The listing builds one solid part. Answer for the finished solid, in the listing's coordinates (mm). A direction names the side the tool comes from. Coordinates: 2 decimals unless noted, no trailing zeros. Write each loop counter-clockwise with the first axis right and the second up, starting at its lowest first coordinate (ties: lowest second). Pieces come first, ordered by that corner, then holes.
```python
from build123d import *

# Parameters (mm, degrees)
SKETCH_1_W          = 31.8
SKETCH_1_H          = 15.8
EXTRUDE_1_DEPTH     = 9.6
SKETCH_2_R          = 2.4
EXTRUDE_4_DEPTH     = 1.7
SKETCH_3_R          = 2.5
CUT_EXTRUDE_1_DEPTH = 1.8


with BuildPart() as part:
    # Эскиз1 → Бобышка-Вытянуть1 (new body)
    with BuildSketch(Plane(origin=(0, 0, 0), x_dir=(1, 0, 0), z_dir=(0, 1, 0))):
        with Locations((15.9, 7.9)):
            Rectangle(SKETCH_1_W, SKETCH_1_H)
    extrude(amount=EXTRUDE_1_DEPTH)

    # Эскиз2 → Бобышка-Вытянуть4 (add)
    with BuildSketch(Plane.XZ):
        with Locations((27.9, -3.9)):
            Circle(SKETCH_2_R)
        with Locations((19.9, -3.9)):
            Circle(SKETCH_2_R)
        with Locations((11.9, -3.9)):
            Circle(SKETCH_2_R)
        with Locations((3.9, -3.9)):
            Circle(SKETCH_2_R)
        with Locations((19.9, -11.9)):
            Circle(SKETCH_2_R)
        with Locations((11.9, -11.9)):
            Circle(SKETCH_2_R)
        with Locations((3.9, -11.9)):
            Circle(SKETCH_2_R)
        with Locations((27.9, -11.9)):
            Circle(SKETCH_2_R)
    extrude(amount=EXTRUDE_4_DEPTH)

    # Эскиз3 → Вырез-Вытянуть1 (cut)
    with BuildSketch(Plane(origin=(0, 9.6, 0), x_dir=(1, 0, 0), z_dir=(0, 1, 0))):
        with Locations((27.9, 3.9)):
            Circle(SKETCH_3_R)
        with Locations((19.9, 3.9)):
            Circle(SKETCH_3_R)
        with Locations((11.9, 3.9)):
            Circle(SKETCH_3_R)
        with Locations((3.9, 3.9)):
            Circle(SKETCH_3_R)
        with Locations((19.9, 11.9)):
            Circle(SKETCH_3_R)
        with Locations((11.9, 11.9)):
            Circle(SKETCH_3_R)
        with Locations((3.9, 11.9)):
            Circle(SKETCH_3_R)
        with Locations((27.9, 11.9)):
            Circle(SKETCH_3_R)
    extrude(amount=-CUT_EXTRUDE_1_DEPTH, mode=Mode.SUBTRACT)


solid = part.part
```
(1) Section C-C, the plane x = 4.5 is taken. Write down the section's boundary in (y, z), plus the area to 3 significant figures.
(2) Section A-A, the plane y = 8.75 is taken. State how many separate pieces and enclosed holes the cut face has, plus the area to 3 significant figures.
(3) Find the intervals of material crossed by probe 1 along Z at (x, y) = (27.9, 9.05); probe 2 along X at (y, z) = (9, -3.9); probe 3 along Z at (x, y) = (4.5, 8), in increasing order.
(4) Which of the six approach directions +Z, -Z, +X, -X, +Y, -Y give full straight-line access (tool end or side, diameter ignored) to faces 1 (the flat face through (28, -1.7, -4)), 2 (the cylindrical face through (9.995, -0.838, -13.36)), 3 (the cylindrical face through (29.24, 8.71, -14.01))?
(5) This flat-tipped pin is pushed along its axis until it touches: pin 1 (1.5 mm diameter, centred on x = 12.5, z = -3, fed in from +Y). Where does it stop, or does it pass through?
(6) Section B-B, the plane x = 27.9 is taken. Write down the section's boundary in (y, z), plus the area to 3 significant figures.
(7) For a pull along Z with two mould halves and no side action, classify faces 4 (the flat face through (16, 5, 0)), 5 (the flat face through (20, -1.7, -12)), 6 (the cylindrical face through (14.285, 8.713, -4.651)) as pulls with the +Z half, pulls with the -Z half, needs draft (parallel to the pull), parting line crosses it, or undercut.
Solution:
1. outline: (-1.7, -14.22) - (0, -14.22) - (0, -15.8) - (9.6, -15.8) - (9.6, -14.33) - (7.8, -14.33) - (7.8, -9.47) - (9.6, -9.47) - (9.6, -6.33) - (7.8, -6.33) - (7.8, -1.47) - (9.6, -1.47) - (9.6, 0) - (0, 0) - (0, -1.58) - (-1.7, -1.58) - (-1.7, -6.22) - (0, -6.22) - (0, -9.58) - (-1.7, -9.58) - close
1. area: 150 mm2
2. separate pieces: 1
2. enclosed holes: 8
2. area: 345 mm2
3. probe 1: z = -15.8 to -14.4, -9.4 to -6.4, -1.4 to 0
3. probe 2: x = 0 to 1.4, 6.4 to 9.4, 14.4 to 17.4, 22.4 to 25.4, 30.4 to 31.8
3. probe 3: z = -15.8 to -14.33, -9.47 to -6.33, -1.47 to 0
4. face 1: +Z, -Z, +X, -X, -Y
4. face 2: -Y
4. face 3: +Y
5. pin 1: stops at y = 7.8
6. outline: (-1.7, -14.3) - (0, -14.3) - (0, -15.8) - (9.6, -15.8) - (9.6, -14.4) - (7.8, -14.4) - (7.8, -9.4) - (9.6, -9.4) - (9.6, -6.4) - (7.8, -6.4) - (7.8, -1.4) - (9.6, -1.4) - (9.6, 0) - (0, 0) - (0, -1.5) - (-1.7, -1.5) - (-1.7, -6.3) - (0, -6.3) - (0, -9.5) - (-1.7, -9.5) - close
6. area: 150 mm2
7. face 4: pulls with the +Z half
7. face 5: needs draft
7. face 6: undercut
